Model file for the job. Use its own axes, mm. A direction names the side the tool comes from. Coordinates: 2 decimals unless noted, no trailing zeros. Loops run counter-clockwise (first coordinate to the right, second up) from the corner with the lowest first, then second, coordinate; pieces in that order, holes last. Notation, with made-up numbers: M 68,3.25 L 122,3.25 A23 ccw 122,25.25 Z; hole C 48.25,-13.5 d8. An arc over 180 degrees is marked long. One line per question, with ' | ' between items. Start each with the question number.
```python
from build123d import *

# Parameters (mm, degrees)
F2_DEPTH = 6.35
F0_R     = 10.9
F3_DEPTH = 12.5
F4_SIZE  = 2
F5_SIZE  = 1
F6_SIZE2 = 1.6454482672
F6_SIZE  = 2.85


with BuildPart() as f2:
    # F1 (on Top) → F2 (new body, symmetric)
    with BuildSketch(Plane.XY):
        with BuildLine():
            Line((-13.9, 36.9362757407), (-13.9, 5.3005428515))
            ThreePointArc((-13.9, 5.3005428515), (-27.8029336636, 3.5865442194), (-38.954053502, 12.0648625736))
            Line((-38.954053502, 12.0648625736), (-38.954053502, -22.4606835239))
            Line((-38.954053502, -22.4606835239), (-25.054053502, -30.4858522656))
            Line((-25.054053502, -30.4858522656), (2.3432948474, -14.667985821))
            ThreePointArc((2.3432948474, -14.667985821), (10.7791280366, -25.8512802448), (9.0122488797, -39.7475924826))
            Line((9.0122488797, -39.7475924826), (38.9122488797, -22.4848194339))
            Line((38.9122488797, -22.4848194339), (38.9122488797, -6.4344819504))
            Line((38.9122488797, -6.4344819504), (11.5149005303, 9.3833844942))
            ThreePointArc((11.5149005303, 9.3833844942), (16.9820010047, 22.2806775501), (29.9, 27.6986714336))
            Line((29.9, 27.6986714336), (0, 44.9614444824))
            Line((0, 44.9614444824), (-13.9, 36.9362757407))
        make_face()
        Polygon((-24.004053502, -27.6279684332), (-35.954053502, -20.7286327163), (-35.954053502, -6.9299612827), (-24.004053502, -0.0306255659), (-12.054053502, -6.9299612827), (-12.054053502, -20.7286327163), align=None, mode=Mode.SUBTRACT)
        with BuildLine():
            ThreePointArc((0, 13.9), (9.8287842585, 9.8287842585), (13.9, 0))
            ThreePointArc((13.9, 0), (13.4287454536, -3.5887038806), (12.0469358931, -6.9340706361))
            Line((12.0469358931, -6.9340706361), (23.9622488797, -0.0547614759))
            Line((23.9622488797, -0.0547614759), (35.9122488797, -6.9540971927))
            Line((35.9122488797, -6.9540971927), (35.9122488797, -20.7527686263))
            Line((35.9122488797, -20.7527686263), (23.9622488797, -27.6521043431))
            Line((23.9622488797, -27.6521043431), (12.0122488797, -20.7527686263))
            Line((12.0122488797, -20.7527686263), (12.0122488797, -6.9939886226))
            ThreePointArc((12.0122488797, -6.9939886226), (-12.0504448435, -6.927970776), (0, 13.9))
        make_face(mode=Mode.SUBTRACT)
        Polygon((11.95, 20.7993357168), (0, 13.9), (-11.95, 20.7993357168), (-11.95, 34.5980071504), (0, 41.4973428673), (11.95, 34.5980071504), align=None, mode=Mode.SUBTRACT)
        with BuildLine():
            ThreePointArc((12.0469358931, -6.9340706361), (13.4287454536, -3.5887038806), (13.9, 0))
            ThreePointArc((13.9, 0), (9.8287842585, 9.8287842585), (0, 13.9))
            ThreePointArc((0, 13.9), (-12.0504448435, -6.927970776), (12.0122488797, -6.9939886226))
            Line((12.0122488797, -6.9939886226), (12.0122488797, -6.9540971927))
            Line((12.0122488797, -6.9540971927), (12.0469358931, -6.9340706361))
        make_face()
    extrude(amount=F2_DEPTH, both=True)

    # F0 (on Top) → F3 (cut, symmetric)
    with BuildSketch(Plane.XY):
        Circle(F0_R)
    extrude(amount=F3_DEPTH, both=True, mode=Mode.SUBTRACT)

    # F4
    f4_edges = [f2.edges().sort_by_distance(p)[0] for p in [
        (14.95, 36.330058, -6.35),
        (14.95, 36.330058, 6.35),
        (-38.954054, -5.19791, 6.35),
        (-38.954054, -5.19791, -6.35),
        (-32.004054, -26.473268, -6.35),
        (-32.004054, -26.473268, 6.35),
        (23.962249, -31.116206, -6.35),
        (23.962249, -31.116206, 6.35),
        (38.912249, -14.459651, 6.35),
        (38.912249, -14.459651, -6.35),
        (-6.95, 40.94886, -6.35),
        (-6.95, 40.94886, 6.35),
    ]]
    chamfer(f4_edges, length=F4_SIZE)

    # F5
    f5_edges = [f2.edges().sort_by_distance(p)[0] for p in [
        (-10.355379, -21.999569, 6.35),
        (-10.355379, -21.999569, -6.35),
        (-13.9, 19.963709, -6.35),
        (-13.9, 19.963709, 6.35),
        (24.213575, 2.051802, 6.35),
        (24.213575, 2.051802, -6.35),
        (15.828699, 21.020998, 6.35),
        (15.828699, 21.020998, -6.35),
        (-26.135368, 3.217595, 6.35),
        (-26.135368, 3.217595, -6.35),
        (10.264865, -24.222651, -6.35),
        (10.264865, -24.222651, 6.35),
    ]]
    chamfer(f5_edges, length=F5_SIZE)

    # F6
    f6_edges = [f2.edges().sort_by_distance(p)[0] for p in [
        (-10.9, 0, 6.35),
        (-10.9, 0, -6.35),
    ]]
    f6_side = f2.faces().sort_by_distance((-10.9, 0, 0))[0]
    chamfer(f6_edges, length=F6_SIZE, length2=F6_SIZE2, reference=f6_side)


solid = f2.part
```
(1) Band-saw the part on B-B on y = 39.5. Write the cut outline in (x, z).
(2) Band-saw the part on A-A on z = 1.75. Give the number of separate pieces and of enclosed holes in the cut face, then the cut area to 3 significant figures.
(3) Two-plate mould, pull along X, no slides. Class faces 6 (the face through (-11.1, 6.5, -6.35)), 7 (the face through (-30.063, -3.529, 0.089)), 8 (the face through (23.75, -31.24, 0.06)), 9 (the face through (10.4, 3.27, 0.05)): pulls with the +X half, pulls with the -X half, needs draft (parallel to the pull), parting line crosses it, or undercut.
(4) Drill centre lines: line 1 (X direction, y = -12.5, z = 1.5); line 2 (Y direction, x = 0, z = -2.25); line 3 (Y direction, x = 19, z = 0.5). Where is each one in solid material? Low to high. Write a range as [from, to].
(5) 3-axis set-ups, long thin cutter, end or side, ignore diameter. For faces 1 (the face through (29.854, -3.456, 0.089)), 2 (the face through (10.526, -24.478, 5.51)), 3 (the face through (-13.9, 21, 0)), 4 (the face through (24.41, 1.37, 5.84)), 5 (the face through (16.84, 22.14, 0.07)): which of +Z, -Z, +X, -X, +Y, -Y reach the whole face in a straight line?
(6) Pin check, flat tips, straight feed: P1, Ø5, axis at x = -28.5, z = -4.5, coming from the +Y side; P2, Ø4, axis at y = 27, z = 0, coming from the -X side; P3, Ø3, axis at x = -3, z = -1, coming from the +Y side. Stop position of each tip, or through.
Computed values:
1) outline: M -9.46,-4.35 L -5.46,-6.35 L -3.46,-6.35 L -3.46,6.35 L -5.46,6.35 L -9.46,4.35 Z; M 3.46,-6.35 L 5.46,-6.35 L 9.46,-4.35 L 9.46,4.35 L 5.46,6.35 L 3.46,6.35 Z
2) separate pieces: 1 | enclosed holes: 4 | area: 1,530 mm^2
3) face 6: needs draft | face 7: undercut | face 8: pulls with the +X half | face 9: undercut
4) line 1: [-38.95, -35.95], [-12.05, 12.01], [35.91, 38.91] | line 2: [-16.02, -10.9], [10.9, 13.9], [41.5, 44.96] | line 3: [-33.98, -24.79], [-2.92, 5.06], [24.02, 33.99]
5) face 1: +Z, -Z | face 2: +Z | face 3: +Z, -Z, +Y | face 4: +Z, +X | face 5: +Z, -Z, +X
6) P1: y = 4.77 | P2: x = -13.9 | P3: y = 44.1
